Geometry: final body of the model. Coordinates: model frame, mm. A direction names the side the tool comes from. Give positions to 0.01 mm unless a question says otherwise; leave off trailing zeros. Write each loop counter-clockwise with the first axis right and the second up, starting at its lowest first coordinate (ties: lowest second). Pieces come first, ordered by that corner, then holes. Notation, with made-up numbers: (-22.5, 42) - (-18.5, 42) arc R28 ccw to (-18.5, 67) - close; hole circle Ø5 at (-26, -30.75). An arc over 180 degrees is marked (long way). One line per question, with ' | ' between items. Start each with the question number.
```python
from build123d import *

# Parameters (mm, degrees)
F1_DEPTH = 63.5
F0_W     = 22.921771
F0_H     = 19.05
F2_DEPTH = 25.4
F3_DEPTH = 9.525
F0_W_2   = 25.4
F0_H_2   = 28.575
F5_R     = 5.08


with BuildPart() as f1:
    # F0 (on Front) → F1 (new body, symmetric)
    with BuildSketch(Plane.XZ):
        Polygon((-109.419321, -19.310768), (-26.869321, -19.310768), (-26.869321, -0.260768), (-45.919321, -0.260768), (-109.419321, -0.260768), align=None)
    extrude(amount=F1_DEPTH, both=True)

    # F0 (on Front) → F2 (join, symmetric)
    with BuildSketch(Plane.XZ):
        with BuildLine():
            Line((-45.919321, -0.260768), (-26.869321, -0.260768))
            Line((-26.869321, -0.260768), (-26.869321, 15.84063))
            ThreePointArc((-26.869321, 15.84063), (-23.12745, 26.077956), (-13.665816, 31.489232))
            Line((-13.665816, 31.489232), (-7.819321, 31.489232))
            Line((-7.819321, 31.489232), (-7.819321, 50.539232))
            Line((-7.819321, 50.539232), (-14.964541, 50.539232))
            ThreePointArc((-14.964541, 50.539232), (-37.055936, 39.090315), (-45.919321, 15.84063))
            Line((-45.919321, 15.84063), (-45.919321, -0.260768))
        make_face()
        with Locations((3.641564, 41.014232)):
            Rectangle(F0_W, F0_H)
    extrude(amount=F2_DEPTH, both=True)

    # F0 (on Front) → F3 (join, symmetric)
    with BuildSketch(Plane.XZ):
        with BuildLine():
            add(Edge.make_bspline(
                [(-109.419321, -0.260768), (-74.719019, 12.0015), (-55.361759, 50.716016), (-14.964541, 50.539232)],
                knots=[0, 0, 0, 0, 107.248988, 107.248988, 107.248988, 107.248988], degree=3))
            Line((-109.419321, -0.260768), (-45.919321, -0.260768))
            Line((-45.919321, -0.260768), (-45.919321, 15.84063))
            ThreePointArc((-45.919321, 15.84063), (-37.055936, 39.090315), (-14.964541, 50.539232))
        make_face()
    extrude(amount=F3_DEPTH, both=True)

    # F0 (on Front) → F4 (revolve)
    with BuildSketch(Plane.XZ):
        with Locations((30.280679, 42.601732)):
            Rectangle(F0_W_2, F0_H_2)
    revolve(axis=Axis((17.580679, 0, 42.601732), (0, 0, -1)))

    # F5
    f5_edges = [f1.edges().sort_by_distance(p)[0] for p in [
        (-109.419321, -63.5, -9.785768),
        (-109.419321, 63.5, -9.785768),
        (-26.869321, -63.5, -9.785768),
        (-26.869321, 63.5, -9.785768),
    ]]
    fillet(f5_edges, radius=F5_R)


solid = f1.part
```
1) First-contact query: pin 1 Ø10.5 at (y, z) = (-17.5, 2.5) entering from +X; pin 2 Ø10 at (x, y) = (-57.5, 24.5) entering from +Z; pin 3 Ø15 at (x, z) = (-4.5, 22) entering from -Y; pin 4 Ø4 at (x, y) = (17.5, -29) entering from +Z. Flat tips, straight axial feed; report the tip coordinate or a pass-through.
2) Reachability of faces 4 (the flat face through (-62, 9.525, 20)), 5 (the flat face through (-9, 0, 31.489)), 6 (the cylindrical face through (-36.82, -17.57, 39.35)) from +Z, -Z, +X, -X, +Y, -Y: full face, straight path, thin tool, end or side. Return the list, or none.
3) Line query: L1, parallel to X at y = 44, z = -11; L2, parallel to Z at x = 30, y = -11; L3, parallel to Z at x = -63, y = 20.5. Output: solid intervals per line, ascending.
4) Section A-A, the plane y = -44. Output: boundary loops of the cut face in (x, z).
5) Pull-direction query (X, two-part tool) for faces 1 (the flat face through (18, 0, 28.314)), 2 (the cylindrical face through (-23.227, -0.356, 25.958)), 3 (the cylindrical face through (-28.318, -61.972, -9.652)); classes: +X half, -X half, draft (parallel to the pull), parting line (faces both ways), or undercut.
6) Section C-C, the plane y = -12.5. Output: boundary loops of the cut face in (x, z) (3 decimals), plus the area to 3 significant figures.
7) Section B-B, the plane x = 21. Output: boundary loops of the cut face in (y, z), plus the area to 3 significant figures.
Answer key:
1) pin 1: x = -26.87 | pin 2: z = -0.26 | pin 3: y = -17.89 | pin 4: through
2) face 4: +Z, -X, +Y | face 5: -Z | face 6: +Z, -X, -Y
3) L1: -109.42 to -26.87 | L2: 28.31 to 56.89 | L3: -19.31 to -0.26
4) outline: (-109.42, -19.31) - (-26.87, -19.31) - (-26.87, -0.26) - (-109.42, -0.26) - close
5) face 1: draft | face 2: undercut | face 3: +X half
6) outline: (-109.419, -19.311) - (-26.869, -19.311) - (-26.869, 15.841) arc R15.875 cw to (-13.666, 31.489) - (-4.531, 31.489) - (-4.531, 28.314) - (39.692, 28.314) - (39.692, 56.889) - (-4.531, 56.889) - (-4.531, 50.539) - (-14.965, 50.539) arc R34.925 ccw to (-45.919, 15.841) - (-45.919, -0.261) - (-109.419, -0.261) - close | area: 4,030 mm^2
7) outline: (-25.17, 28.31) - (25.17, 28.31) - (25.17, 56.89) - (-25.17, 56.89) - close | area: 1,440 mm^2
